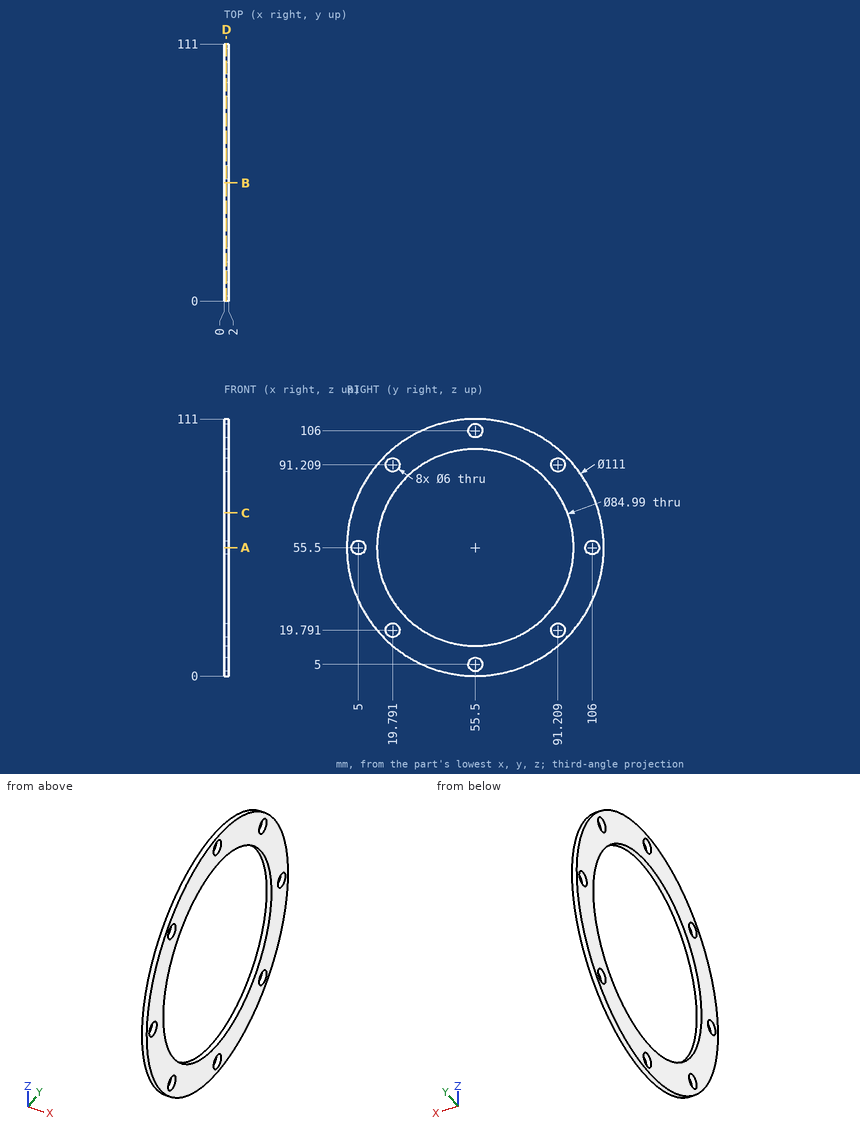
Geometry: see drawing. Coordinates: mm, zero at the bounding-box minimum. Give positions to 0.01 mm unless a question says otherwise; leave off trailing zeros. Loops run counter-clockwise (first coordinate to the right, second up) from the corner with the lowest first, then second, coordinate; pieces in that order, holes last. Notation, with made-up numbers: M 48.5,-2.5 L 101.5,-2.5 A12 cw 101.5,6.5 Z; hole C -10,16.25 d2. An arc over 180 degrees is marked long. Use one line per item in the form item = value.
1. Line query: L1, parallel to Y at x = 0.4, z = 55.5 (3 decimals); L2, parallel to Z at x = 1, y = 90 (1 decimal); L3, parallel to Y at x = 1.35, z = 20. Output: solid intervals per line, ascending.
Numbers:
L1 = 0 to 2, 8 to 13.005, 97.995 to 103, 109 to 111
L2 = 12 to 17, 22.5 to 30.7, 80.3 to 88.5, 94 to 99
L3 = 12.84 to 16.8, 22.78 to 32.14, 78.86 to 88.22, 94.2 to 98.16
2. First-contact query: pin 1 (9.5 mm diameter, centred on y = 91.21, z = 91.21, fed in from -X). Flat tip, straight axial feed; report the tip coordinate or a pass-through.
Numbers:
pin_1 = 0
3. Section query D-D, the plane x = 0.9. Count the separate pieces of the cut face and the enclosed holes in it, and give its area (3 significant figures).
Numbers:
separate_pieces = 1
enclosed_holes = 9
area = 3,780 mm²
4. Section query B-B, the plane y = 51. Return the cut outline in (x, z).
Numbers:
outline = M 0,0.18 L 2,0.18 L 2,13.24 L 0,13.24 Z; M 0,97.76 L 2,97.76 L 2,110.82 L 0,110.82 Z
5. Section query C-C, the plane z = 70.5. Return the cut outline in (x, y).
Numbers:
outline = M 0,2.07 L 2,2.07 L 2,15.74 L 0,15.74 Z; M 0,95.26 L 2,95.26 L 2,108.93 L 0,108.93 Z
6. Section query A-A, the plane z = 55.5. Return the cut outline in (x, y) (3 decimals).
Numbers:
outline = M 0,0 L 2,0 L 2,2 L 0,2 Z; M 0,8 L 2,8 L 2,13.005 L 0,13.005 Z; M 0,97.995 L 2,97.995 L 2,103 L 0,103 Z; M 0,109 L 2,109 L 2,111 L 0,111 Z
